from build123d import *

# Parameters (mm, degrees)
CYLINDER_R     = 0.25
CYLINDER_DEPTH = 6
ARRAY_X_COUNT  = 4
ARRAY_X_PITCH  = 1.8
BOX011_W       = 7
BOX011_H       = 7
BOX011_DEPTH   = 3
BOX010_W       = 0.5
BOX010_H       = 4
BOX010_DEPTH   = 10
BOX009_W       = 0.5
BOX009_H       = 4
BOX009_DEPTH   = 10
BOX008_W       = 8
BOX008_H       = 3
BOX008_DEPTH   = 10
BOX007_W       = 9
BOX007_H       = 3
BOX007_DEPTH   = 10
BOX006_W       = 0.4
BOX006_H       = 10
BOX006_DEPTH   = 1
BOX005_W       = 0.4
BOX005_H       = 10
BOX005_DEPTH   = 1
BOX004_W       = 0.4
BOX004_H       = 10
BOX004_DEPTH   = 1
BOX003_W       = 0.4
BOX003_H       = 10
BOX003_DEPTH   = 1
BOX002_W       = 10
BOX002_H       = 5
BOX002_DEPTH   = 6.5
BOX001_W       = 10
BOX001_H       = 4
BOX001_DEPTH   = 1


with BuildPart() as array:
    # Cylinder → Cylinder (new body)
    with BuildSketch(Plane(origin=(2, 2, -2), x_dir=(1, 0, 0), z_dir=(0, 0, 1))):
        Circle(CYLINDER_R)
    extrude(amount=CYLINDER_DEPTH)

    # Array X: Array ×4


with BuildPart() as array_1:
    add(array.part)
    with Locations(*[(i * ARRAY_X_PITCH, 0, 0) for i in range(1, ARRAY_X_COUNT)]):
        add(array.part)


with BuildPart() as cubo011:
    # Box011 → Box011 (new body)
    with BuildSketch(Plane(origin=(1.5, 3, 4.5), x_dir=(1, 0, 0), z_dir=(0, 0, 1))):
        with Locations((3.5, 3.5)):
            Rectangle(BOX011_W, BOX011_H)
    extrude(amount=BOX011_DEPTH)


with BuildPart() as cubo010:
    # Box010 → Box010 (new body)
    with BuildSketch(Plane(origin=(9.25, 0.5, 1.1), x_dir=(1, 0, 0), z_dir=(0, 0, 1))):
        with Locations((0.25, 2)):
            Rectangle(BOX010_W, BOX010_H)
    extrude(amount=BOX010_DEPTH)


with BuildPart() as cubo009:
    # Box009 → Box009 (new body)
    with BuildSketch(Plane(origin=(0.25, 0.5, 1.1), x_dir=(1, 0, 0), z_dir=(0, 0, 1))):
        with Locations((0.25, 2)):
            Rectangle(BOX009_W, BOX009_H)
    extrude(amount=BOX009_DEPTH)


with BuildPart() as cubo008:
    # Box008 → Box008 (new body)
    with BuildSketch(Plane(origin=(1, 4, 0), x_dir=(1, 0, 0), z_dir=(0, 0, 1))):
        with Locations((4, 1.5)):
            Rectangle(BOX008_W, BOX008_H)
    extrude(amount=BOX008_DEPTH)


with BuildPart() as cubo007:
    # Box007 → Box007 (new body)
    with BuildSketch(Plane(origin=(0.5, 0.5, 1.1), x_dir=(1, 0, 0), z_dir=(0, 0, 1))):
        with Locations((4.5, 1.5)):
            Rectangle(BOX007_W, BOX007_H)
    extrude(amount=BOX007_DEPTH)


with BuildPart() as cubo006:
    # Box006 → Box006 (new body)
    with BuildSketch(Plane(origin=(7.2, -3, 0), x_dir=(1, 0, 0), z_dir=(0, 0, 1))):
        with Locations((0.2, 5)):
            Rectangle(BOX006_W, BOX006_H)
    extrude(amount=BOX006_DEPTH)


with BuildPart() as cubo005:
    # Box005 → Box005 (new body)
    with BuildSketch(Plane(origin=(5.4, -3, 0), x_dir=(1, 0, 0), z_dir=(0, 0, 1))):
        with Locations((0.2, 5)):
            Rectangle(BOX005_W, BOX005_H)
    extrude(amount=BOX005_DEPTH)


with BuildPart() as cubo004:
    # Box004 → Box004 (new body)
    with BuildSketch(Plane(origin=(3.6, -3, 0), x_dir=(1, 0, 0), z_dir=(0, 0, 1))):
        with Locations((0.2, 5)):
            Rectangle(BOX004_W, BOX004_H)
    extrude(amount=BOX004_DEPTH)


with BuildPart() as cubo003:
    # Box003 → Box003 (new body)
    with BuildSketch(Plane(origin=(1.8, -3, 0), x_dir=(1, 0, 0), z_dir=(0, 0, 1))):
        with Locations((0.2, 5)):
            Rectangle(BOX003_W, BOX003_H)
    extrude(amount=BOX003_DEPTH)


with BuildPart() as cubo002:
    # Box002 → Box002 (new body)
    with BuildSketch(Plane.XY.offset(1)):
        with Locations((5, 2.5)):
            Rectangle(BOX002_W, BOX002_H)
    extrude(amount=BOX002_DEPTH)


with BuildPart() as conector:
    # Box001 → Box001 (new body)
    with BuildSketch(Plane.XY):
        with Locations((5, 2)):
            Rectangle(BOX001_W, BOX001_H)
    extrude(amount=BOX001_DEPTH)

    # Fusion: union Cubo002
    add(cubo002.part)

    # Cut: cut Cubo003
    add(cubo003.part, mode=Mode.SUBTRACT)

    # Cut001: cut Cubo004
    add(cubo004.part, mode=Mode.SUBTRACT)

    # Cut002: cut Cubo005
    add(cubo005.part, mode=Mode.SUBTRACT)

    # Cut003: cut Cubo006
    add(cubo006.part, mode=Mode.SUBTRACT)

    # Cut004: cut Cubo007
    add(cubo007.part, mode=Mode.SUBTRACT)

    # Cut005: cut Cubo008
    add(cubo008.part, mode=Mode.SUBTRACT)

    # Cut006: cut Cubo009
    add(cubo009.part, mode=Mode.SUBTRACT)

    # Cut007: cut Cubo010
    add(cubo010.part, mode=Mode.SUBTRACT)

    # Cut008: cut Cubo011
    add(cubo011.part, mode=Mode.SUBTRACT)

    # Fusion001: union Array
    add(array_1.part)


with BuildPart() as conector_1:
    # Fusion001 placement: moved
    add(conector.part.moved(Location((5, 13.5, 1.5))))


solid = conector_1.part
Geometry check sheet. Reference: the model listing, model coordinates, mm. A direction names the side the tool comes from. Give positions to 0.01 mm unless a question says otherwise; leave off trailing zeros. Order: outer loops, then holes, each group sorted by start corner. A loop starts at its lowest first (then second) coordinate and runs counter-clockwise, first axis right, second up. Notation, with made-up numbers: M 8,-7 L 52,-7 A26 ccw 52,16 Z; hole C 24.5,84.5 d1. An arc over 180 degrees is marked long. Use a Markdown table: item, result.
Item 1: Section check B-B (z = 4.25). Record the cut outline in (x, y), and give its area (3 significant figures).
Answers follow:
| item | result |
|---|---|
| outline | M 5,13.5 L 15,13.5 L 15,18.5 L 14,18.5 L 14,17.5 L 6,17.5 L 6,18.5 L 5,18.5 Z; C 7,15.5 d0.5; C 8.8,15.5 d0.5; C 10.6,15.5 d0.5; C 12.4,15.5 d0.5; hole M 5.25,14 L 14.75,14 L 14.75,18 L 14.25,18 L 14.25,17 L 5.75,17 L 5.75,18 L 5.25,18 Z |
| area | 13.3 mm2 |
Item 2: Material ranges on line 1 along X through (y, z) = (17.75, 5.75); line 2 along X through (y, z) = (16.5, 6.5); line 3 along X through (y, z) = (18.2, 6), recorded low to high.
Answers follow:
| item | result |
|---|---|
| line 1 | x = 5 to 5.25, 5.75 to 6, 14 to 14.25, 14.75 to 15 |
| line 2 | x = 5 to 5.25, 14.75 to 15 |
| line 3 | x = 5 to 6, 14 to 15 |
Item 3: Tool access check on faces 4 (the flat face through (5.49, 18.12, 2.5)), 5 (the flat face through (6, 18, 6)), 6 (the flat face through (10, 17, 5)), 7 (the flat face through (10.8, 14, 2)). Record the directions out of +Z, -Z, +X, -X, +Y, -Y that give a thin tool (end or side, any length) a straight path to the whole face; none if there is none.
Answers follow:
| item | result |
|---|---|
| face 4 | -Z, +X, -X, +Y |
| face 5 | +Z, -Z, +Y |
| face 6 | +Z |
| face 7 | -Z, -Y |
Item 4: Section check D-D (z = 5.75). Record the cut outline in (x, y).
Answers follow:
| item | result |
|---|---|
| outline | M 5,13.5 L 15,13.5 L 15,18.5 L 14,18.5 L 14,17.5 L 6,17.5 L 6,18.5 L 5,18.5 Z; hole M 5.25,14 L 14.75,14 L 14.75,18 L 14.25,18 L 14.25,17 L 5.75,17 L 5.75,18 L 5.25,18 Z |
Item 5: Section check C-C (x = 7). Record the cut outline in (y, z), and give its area (3 significant figures).
Answers follow:
| item | result |
|---|---|
| outline | M 13.5,2.5 L 15.25,2.5 L 15.25,-0.5 L 15.75,-0.5 L 15.75,2.5 L 17.5,2.5 L 17.5,6 L 17,6 L 17,2.6 L 15.75,2.6 L 15.75,5.5 L 15.25,5.5 L 15.25,2.6 L 14,2.6 L 14,9 L 13.5,9 Z |
| area | 8.25 mm2 |
Item 6: Section check A-A (y = 17.7). Record the cut outline in (x, z), and give its area (3 significant figures).
Answers follow:
| item | result |
|---|---|
| outline | M 5,2.5 L 6,2.5 L 6,9 L 5.75,9 L 5.75,2.6 L 5.25,2.6 L 5.25,9 L 5,9 Z; M 14,2.5 L 15,2.5 L 15,9 L 14.75,9 L 14.75,2.6 L 14.25,2.6 L 14.25,9 L 14,9 Z |
| area | 6.60 mm2 |
Item 7: Draft check along Y on faces 1 (the flat face through (5.5, 18.5, 5.7)), 2 (the flat face through (12.2, 17, 2)), 3 (the flat face through (14.25, 17.5, 5.8)). Enter one of: +Y half, -Y half, draft (parallel to the pull), parting line (faces both ways), or undercut.
Answers follow:
| item | result |
|---|---|
| face 1 | +Y half |
| face 2 | draft |
| face 3 | undercut |
Item 8: Depth check by flat-ended pin: P1, Ø1.1, axis at x = 14.5, y = 18, coming from the -Z side; P2, Ø2, axis at x = 9.5, y = 15.5, coming from the +Z side; P3, Ø1.5, axis at x = 7.5, z = 2.5, coming from the +Y side. Enter the tip coordinate at first touch or a pass-through.
Answers follow:
| item | result |
|---|---|
| P1 | stops at z = 1.5 |
| P2 | stops at z = 5.5 |
| P3 | stops at y = 17.5 |
